from build123d import *

# Parameters (mm, degrees)
F1_DEPTH = 15
F2_DEPTH = 7.5
F3_DEPTH = 15


with BuildPart() as f1:
    # F0 (on Front) → F1 (new body, symmetric)
    with BuildSketch(Plane.XZ):
        Polygon((40, 15), (0, 0), (40, 0), align=None)
        Polygon((30, 18.75), (10, 26.25), (10, 18.75), align=None)
        Polygon((0, 30), (0, 0), (40, 15), (30, 18.75), (10, 18.75), (10, 26.25), align=None)
    extrude(amount=F1_DEPTH, both=True)

    # F0 (on Front) → F2 (join, symmetric)
    with BuildSketch(Plane.XZ):
        Polygon((30, 26.25), (10, 26.25), (30, 18.75), align=None)
    extrude(amount=F2_DEPTH, both=True)

    # F0 (on Front) → F3 (cut, symmetric)
    with BuildSketch(Plane.XZ):
        Polygon((40, 15), (0, 0), (40, 0), align=None)
    extrude(amount=F3_DEPTH, both=True, mode=Mode.SUBTRACT)


solid = f1.part
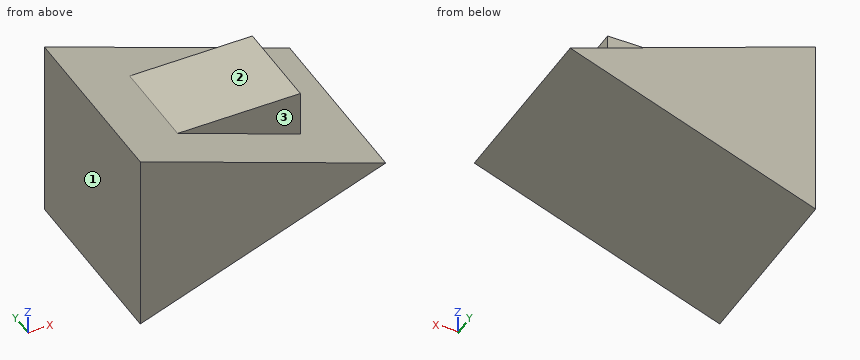
Read the model definition and answer for the solid it produces. Units are mm, in the model's axes. Face numbers are marked on the shaded views. A direction names the side the tool comes from. Give positions to 0.01 mm unless a question says otherwise; leave off trailing zeros. Loops run counter-clockwise (first coordinate to the right, second up) from the corner with the lowest first, then second, coordinate; pieces in that order, holes last. Notation, with made-up numbers: (66, 14.5) -> (121, 14.5) arc R16 cw to (121, 29.5) -> close; hole circle Ø8 at (29, 35.25). An arc over 180 degrees is marked (long way). Answer as CSV lines item,"result".
Item 1: Find section B-B on x = 29. Give the vertices of the cut face in (y, z) (3 decimals), plus the area to 3 significant figures.
Returned:
outline,"(-15, 10.875) -> (15, 10.875) -> (15, 19.125) -> (7.5, 19.125) -> (7.5, 26.25) -> (-7.5, 26.25) -> (-7.5, 19.125) -> (-15, 19.125) -> close"
area,"354 mm²"
Item 2: Consider line 1 (X direction, y = 5.75, z = 23.5); line 2 (Z direction, x = 19.5, y = 13.25); line 3 (Z direction, x = 12.5, y = 5.5). Determine where each line is inside the solid, lowest interval first. Write a range as [from, to].
Returned:
line 1,"x = [0, 30]"
line 2,"z = [7.31, 22.69]"
line 3,"z = [4.69, 26.25]"
Item 3: Each of these flat-tipped pins is pushed along its axis until it touches: pin 1 (3 mm diameter, centred on y = -7, z = 24, fed in from +X); pin 2 (12 mm diameter, centred on y = 3, z = 18, fed in from -X); pin 3 (3 mm diameter, centred on x = 32.5, y = -8, fed in from -Z) (3 decimals); pin 4 (2 mm diameter, centred on x = 22, z = 23, fed in from +Y). Where does it stop, or does it pass through?
Returned:
pin 1,"stops at x = 30"
pin 2,"stops at x = 0"
pin 3,"stops at z = 11.625"
pin 4,"stops at y = 7.5"
Item 4: Find section A-A on z = 25.5. Give the vertices of the cut face in (x, y), plus the area to 3 significant figures.
Returned:
outline,"(0, -15) -> (12, -15) -> (12, -7.5) -> (30, -7.5) -> (30, 7.5) -> (12, 7.5) -> (12, 15) -> (0, 15) -> close"
area,"630 mm²"
Item 5: For the marked faces 1, 2 and 3, determine the directions among +Z, -Z, +X, -X, +Y, -Y from which every point of the face is accessible in a straight line to the end or side of a thin tool.
Returned:
face 1,"+Z, -Z, -X, +Y, -Y"
face 2,"+Z, +X, +Y, -Y"
face 3,"+Z, +X, -Y"
Item 6: Find section C-C on y = 0. Give the vertices of the cut face in (x, z).
Returned:
outline,"(0, 0) -> (40, 15) -> (30, 18.75) -> (30, 26.25) -> (10, 26.25) -> (0, 30) -> close"
Item 7: Find section D-D on z = 6. Give the vertices of the cut face in (x, y), plus the area to 3 significant figures.
Returned:
outline,"(0, -15) -> (16, -15) -> (16, 15) -> (0, 15) -> close"
area,"480 mm²"
